Here's how the part is built. I have some questions about the finished solid (model axes, mm). Face numbers are marked on the shaded views. A direction names the side the tool comes from. Round coordinates to 2 decimals unless told otherwise and drop trailing zeros. Write each loop counter-clockwise with the first axis right and the second up, starting at its lowest first coordinate (ties: lowest second). Pieces come first, ordered by that corner, then holes. Notation, with made-up numbers: (72.5, 14.25) - (123.5, 14.25) arc R15 cw to (123.5, 21.25) - close; hole circle Ø11 at (48.25, 21). An arc over 180 degrees is marked (long way). One line per item, written item: value. Start each with the question number.
Item 1: Imagine slicing it at B-B, the plane z = 40.5. Please give me the cut outline in (x, y), then the cut area to 3 significant figures.
Item 2: Imagine slicing it at D-D, the plane z = 10. Please give me the cut outline in (x, y), then the cut area to 3 significant figures.
Item 3: Imagine slicing it at C-C, the plane y = 2. Please give me the cut outline in (x, z), then the cut area to 3 significant figures.
Item 4: If I drill on line 1 (X direction, y = -3.5, z = 14); line 2 (Y direction, x = -30, z = 1); line 3 (X direction, y = -13, z = 33), over which ranges is the centre line in solid material (lowest first)?
Item 5: For P1, Ø8, axis at x = -16.5, z = 4.5, coming from the -Y side; P2, Ø2.5, axis at x = -30, y = -25.99, coming from the +Z side; P3, Ø1, axis at x = 30, z = 1, coming from the +Y side, each with a flat end and sliding along its axis, tell me the tip position at first contact or that it passes through.
Item 6: Imagine slicing it at A-A, the plane x = -30. Please give me the cut outline in (y, z), then the cut area to 3 significant figures.
Item 7: For the marked faces 1, 2, 3, 4 and 5, which set-ups out of +Z, -Z, +X, -X, +Y, -Y let a thin tool reach every point of the face, with its end or its side?
```python
from build123d import *

# Parameters (mm, degrees)
ESQUISSE1_W        = 55
ESQUISSE1_H        = 68
BOSS_EXTRU_1_DEPTH = 25
ESQUISSE3_R        = 1.5
BOSS_EXTRU_2_DEPTH = 20
BOSS_EXTRU_3_START = -5
ESQUISSE4_R        = 28.5
BOSS_EXTRU_3_DEPTH = 15
ESQUISSE5_W        = 5
ESQUISSE5_H        = 5
BOSS_EXTRU_4_DEPTH = 2


with BuildPart() as part:
    # Esquisse1 → Boss.-Extru.1 (new body)
    with BuildSketch(Plane.XY):
        Rectangle(ESQUISSE1_W, ESQUISSE1_H)
    extrude(amount=BOSS_EXTRU_1_DEPTH)

    # Esquisse3 → Boss.-Extru.2 (add)
    with BuildSketch(Plane.ZY.offset(27.5)):
        with Locations((15, -24)):
            Circle(ESQUISSE3_R)
    boss_extru_2 = extrude(amount=BOSS_EXTRU_2_DEPTH)

    # Symétrie1: Boss.-Extru.2 across plane
    add(boss_extru_2.mirror(Plane(origin=(0, 0, 0), x_dir=(0, 0, 1), z_dir=(1, 0, 0))))

    # Esquisse4 → Boss.-Extru.3 (add)
    with BuildSketch(Plane.ZY.offset(47.5).offset(BOSS_EXTRU_3_START)):
        with Locations((15, -24)):
            Circle(ESQUISSE4_R)
    boss_extru_3 = extrude(amount=BOSS_EXTRU_3_DEPTH)

    # Symétrie2: Boss.-Extru.3 across plane
    add(boss_extru_3.mirror(Plane(origin=(0, 0, 0), x_dir=(0, 0, 1), z_dir=(1, 0, 0))))

    # Esquisse5 → Boss.-Extru.4 (add)
    with BuildSketch(Plane(origin=(0, 0, 0), x_dir=(-1, 0, 0), z_dir=(0, 0, -1))):
        with Locations((30, -25.993461036)):
            Rectangle(ESQUISSE5_W, ESQUISSE5_H)
    boss_extru_4 = extrude(amount=-BOSS_EXTRU_4_DEPTH)

    # Esquisse9 → Dégagement M31 (revolve, cut)
    with BuildSketch(Plane(origin=(-30, -25.993461036, 0), x_dir=(0, 1, 0), z_dir=(1, 0, 0))):
        Polygon((0, 0), (0, 4.021463052), (1.7, 3), (1.7, 0), align=None)
    d_gagement_m31 = revolve(axis=Axis((-30, -25.993461036, -6.35), (0, 0, 1)), mode=Mode.SUBTRACT)

    # Symétrie3: Boss.-Extru.4, Dégagement M31 across plane
    add(boss_extru_4.mirror(Plane(origin=(0, 0, 0), x_dir=(0, 0, 1), z_dir=(1, 0, 0))))
    add(d_gagement_m31.mirror(Plane(origin=(0, 0, 0), x_dir=(0, 0, 1), z_dir=(1, 0, 0))), mode=Mode.SUBTRACT)


solid = part.part
```
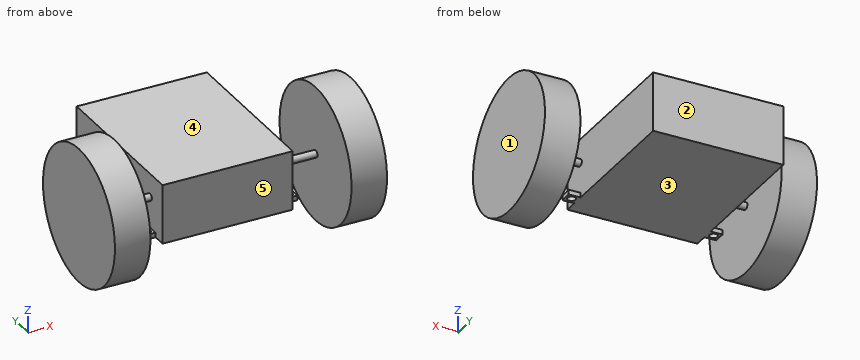
Values follow:
1. outline: (-57.5, -36.73) - (-42.5, -36.73) - (-42.5, -11.27) - (-57.5, -11.27) - close; (42.5, -36.73) - (57.5, -36.73) - (57.5, -11.27) - (42.5, -11.27) - close
1. area: 764 mm^2
2. outline: (-57.5, -52.06) - (-42.5, -52.06) - (-42.5, 4.06) - (-57.5, 4.06) - close; (-27.5, -34) - (27.5, -34) - (27.5, 34) - (-27.5, 34) - close; (42.5, -52.06) - (57.5, -52.06) - (57.5, 4.06) - (42.5, 4.06) - close
2. area: 5,420 mm^2
3. outline: (-57.5, 3.33) - (-42.5, 3.33) - (-42.5, 26.67) - (-57.5, 26.67) - close; (-27.5, 0) - (27.5, 0) - (27.5, 25) - (-27.5, 25) - close; (42.5, 3.33) - (57.5, 3.33) - (57.5, 26.67) - (42.5, 26.67) - close
3. area: 2,080 mm^2
4. line 1: x = -57.5 to -42.5, -27.5 to 27.5, 42.5 to 57.5
4. line 2: y = -28.49 to -27.69, -24.29 to -23.49
4. line 3: x = -57.5 to -42.5, 42.5 to 57.5
5. P1: stops at y = -34
5. P2: stops at z = 16.3
5. P3: stops at y = -23.49
6. outline: (-28.49, 0) - (-27.69, 0) - (-27.69, 2) - (-28.49, 2) - close; circle Ø3 at (-24, 15); (-24.29, 0) - (-23.49, 0) - (-23.49, 2) - (-24.29, 2) - close
6. area: 10.3 mm^2
7. face 1: +Z, -Z, +X, +Y, -Y
7. face 2: +Z, -Z, +X, -X, +Y
7. face 3: -Z, +Y, -Y
7. face 4: +Z, +Y, -Y
7. face 5: +Z, -Z, -Y
